from build123d import *

# Parameters (mm, degrees)
ESQUISSE1_R                  = 11.1
ESQUISSE1_R_2                = 1.65
ESQUISSE1_R_3                = 2.65
ESQUISSE1_W                  = 8.6
ESQUISSE1_H                  = 4.6
ESQUISSE1_W_2                = 4.6
ESQUISSE1_H_2                = 8.6
BOSS_EXTRU_1_DEPTH           = 16
ENL_V_MAT_EXTRU_3_DEPTH      = 10
CHANFREIN1_SIZE              = 2
ESQUISSE6_R                  = 2.6
ENL_V_MAT_EXTRU_4_DEPTH      = 17
R_P_TITION_CIRCULAIRE1_COUNT = 4


with BuildPart() as part:
    # Esquisse1 → Boss.-Extru.1 (new body)
    with BuildSketch(Plane.XY):
        with BuildLine():
            Line((-6.105930323, 29.167749568), (-6.105930323, 23.762922109))
            Line((-6.105930323, 23.762922109), (6.105930323, 23.762922109))
            Line((6.105930323, 23.762922109), (6.105930323, 29.167749568))
            ThreePointArc((6.105930323, 29.167749568), (21.071782079, 21.071782079), (29.167749568, 6.105930323))
            Line((29.167749568, 6.105930323), (23.762922109, 6.105930323))
            Line((23.762922109, 6.105930323), (23.762922109, -6.105930323))
            Line((23.762922109, -6.105930323), (29.167749568, -6.105930323))
            ThreePointArc((29.167749568, -6.105930323), (21.071782079, -21.071782079), (6.105930323, -29.167749568))
            Line((6.105930323, -29.167749568), (6.105930323, -23.762922109))
            Line((6.105930323, -23.762922109), (-6.105930323, -23.762922109))
            Line((-6.105930323, -23.762922109), (-6.105930323, -29.167749568))
            ThreePointArc((-6.105930323, -29.167749568), (-21.071782079, -21.071782079), (-29.167749568, -6.105930323))
            Line((-29.167749568, -6.105930323), (-23.762922109, -6.105930323))
            Line((-23.762922109, -6.105930323), (-23.762922109, 6.105930323))
            Line((-23.762922109, 6.105930323), (-29.167749568, 6.105930323))
            ThreePointArc((-29.167749568, 6.105930323), (-21.071782079, 21.071782079), (-6.105930323, 29.167749568))
        make_face()
        Circle(ESQUISSE1_R, mode=Mode.SUBTRACT)
        with Locations((-10.960155108, 18.983545507)):
            Circle(ESQUISSE1_R_2, mode=Mode.SUBTRACT)
        with Locations((18.983545507, 10.960155108)):
            Circle(ESQUISSE1_R_2, mode=Mode.SUBTRACT)
        with Locations((10.960155108, -18.983545507)):
            Circle(ESQUISSE1_R_2, mode=Mode.SUBTRACT)
        with Locations((-18.983545507, -10.960155108)):
            Circle(ESQUISSE1_R_2, mode=Mode.SUBTRACT)
        with Locations((-13.925584753, 9.750799418)):
            Circle(ESQUISSE1_R_3, mode=Mode.SUBTRACT)
        with Locations((9.750799418, 13.925584753)):
            Circle(ESQUISSE1_R_3, mode=Mode.SUBTRACT)
        with Locations((13.925584753, -9.750799418)):
            Circle(ESQUISSE1_R_3, mode=Mode.SUBTRACT)
        with Locations((-9.750799418, -13.925584753)):
            Circle(ESQUISSE1_R_3, mode=Mode.SUBTRACT)
        with Locations((0, 16.762922109)):
            Rectangle(ESQUISSE1_W, ESQUISSE1_H, mode=Mode.SUBTRACT)
        with Locations((16.762922109, 0)):
            Rectangle(ESQUISSE1_W_2, ESQUISSE1_H_2, mode=Mode.SUBTRACT)
        with Locations((0, -16.762922109)):
            Rectangle(ESQUISSE1_W, ESQUISSE1_H, mode=Mode.SUBTRACT)
        with Locations((-16.762922109, 0)):
            Rectangle(ESQUISSE1_W_2, ESQUISSE1_H_2, mode=Mode.SUBTRACT)
    extrude(amount=BOSS_EXTRU_1_DEPTH)

    # Esquisse5 → Enlèv. mat.-Extru.3 (cut)
    with BuildSketch(Plane(origin=(0, 0, 0), x_dir=(-1, 0, 0), z_dir=(0, 0, -1))):
        Polygon((9.191312546, 9.750799418), (11.558448649, 5.650799418), (16.292720857, 5.650799418), (18.65985696, 9.750799418), (16.292720857, 13.850799418), (11.558448649, 13.850799418), align=None)
        Polygon((-9.750799418, 9.191312546), (-5.650799418, 11.558448649), (-5.650799418, 16.292720857), (-9.750799418, 18.65985696), (-13.850799418, 16.292720857), (-13.850799418, 11.558448649), align=None)
        Polygon((9.750799418, -9.191312546), (5.650799418, -11.558448649), (5.650799418, -16.292720857), (9.750799418, -18.65985696), (13.850799418, -16.292720857), (13.850799418, -11.558448649), align=None)
        Polygon((-9.191312546, -9.750799418), (-11.558448649, -5.650799418), (-16.292720857, -5.650799418), (-18.65985696, -9.750799418), (-16.292720857, -13.850799418), (-11.558448649, -13.850799418), align=None)
    extrude(amount=-ENL_V_MAT_EXTRU_3_DEPTH, mode=Mode.SUBTRACT)

    # Chanfrein1
    chanfrein1_edges = [part.edges().sort_by_distance(p)[0] for p in [
        (-12.610155108, 18.983545507, 16),
        (17.333545507, 10.960155108, 16),
        (9.310155108, -18.983545507, 16),
        (-20.633545507, -10.960155108, 16),
    ]]
    chamfer(chanfrein1_edges, length=CHANFREIN1_SIZE)

    # Esquisse6 → Enlèv. mat.-Extru.4 (cut)
    with BuildSketch(Plane.ZY.offset(23.762922109)):
        with Locations((10, 0)):
            Circle(ESQUISSE6_R)
    enl_v_mat_extru_4 = extrude(amount=-ENL_V_MAT_EXTRU_4_DEPTH, mode=Mode.SUBTRACT)

    # Répétition circulaire1: Enlèv. mat.-Extru.4 ×4 about axis
    r_p_tition_circulaire1_axis = Axis((0, 0, 0), (0, 0, 1))
    for i in range(1, R_P_TITION_CIRCULAIRE1_COUNT):
        add(enl_v_mat_extru_4.rotate(r_p_tition_circulaire1_axis, i * 360 / R_P_TITION_CIRCULAIRE1_COUNT), mode=Mode.SUBTRACT)


solid = part.part
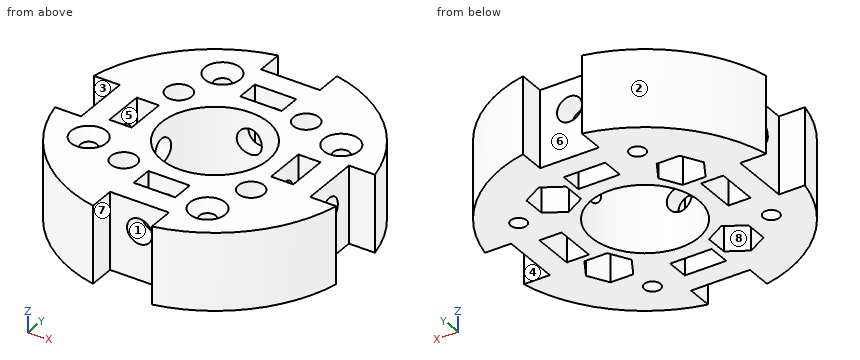
Design review of the part built by this model. Coordinates are the model's own, in mm. Face numbers are marked on the shaded views. A direction names the side the tool comes from. Give positions to 0.01 mm unless a question says otherwise; leave off trailing zeros. Loops run counter-clockwise (first coordinate to the right, second up) from the corner with the lowest first, then second, coordinate; pieces in that order, holes last. Notation, with made-up numbers: M -22,-5.75 L 35,-5.75 A20 cw 35,-0.75 Z; hole C -23,33 d5. An arc over 180 degrees is marked long. Answer as a JSON object with one key per item and string values.
Item 1: Mouldability with a two-part tool opening along X and no side actions: class the marked faces 1, 2 and 3 as pulls with the +X half, pulls with the -X half, needs draft (parallel to the pull), parting line crosses it, or undercut.
Output values:
{"face 1": "undercut", "face 2": "pulls with the -X half", "face 3": "needs draft"}
Item 2: We need section A-A (y = 0). Count the separate pieces of the cut face and the enclosed holes in it, and give its area (3 significant figures).
Output values:
{"separate pieces": "8", "enclosed holes": "0", "area": "174 mm2"}
Item 3: Machinability: for the marked faces 4, 5, 6, 7 and 8, which of the approach directions +Z, -Z, +X, -X, +Y, -Y give a long, thin tool a straight path to every point of the face, cutting with its end or side? Answer none if there is none.
Output values:
{"face 4": "+Z, -Z, +X", "face 5": "+Z, -Z", "face 6": "+Z, -Z, +Y", "face 7": "+Z, -Z, -Y", "face 8": "-Z"}
Item 4: Wall thickness on line 1 along Y through (x, z) = (-12, 13.5); line 2 along Z through (x, y) = (-12.85, 0); line 3 along Y through (x, z) = (3.5, 15.25): over which ranges is each line inside the solid? List them lowest first.
Output values:
{"line 1": "y = -27.28 to -15.33, -12.52 to 7.93, 11.57 to 17.7, 20.26 to 27.28", "line 2": "z = 0 to 7.4, 12.6 to 16", "line 3": "y = -23.76 to -19.06, -14.46 to -10.53, 10.53 to 14.46, 19.06 to 23.76"}
Item 5: We need section C-C (y = -24.5). State the section outline as (x, z) points.
Output values:
{"outline": "M -16.96,0 L -6.11,0 L -6.11,16 L -16.96,16 Z; M 6.11,0 L 16.96,0 L 16.96,16 L 6.11,16 Z"}
Item 6: For P1, Ø8.5, axis at x = 0, z = 10, coming from the -Y side; P2, Ø2.5, axis at x = 1.5, z = 8.5, coming from the +Y side; P3, Ø1, axis at x = -21, z = 12, coming from the -Y side, all flat-tipped, find the tip position at first contact; note any pin that passes through.
Output values:
{"P1": "stops at y = -23.76", "P2": "stops at y = 23.76", "P3": "stops at y = -21.63"}
